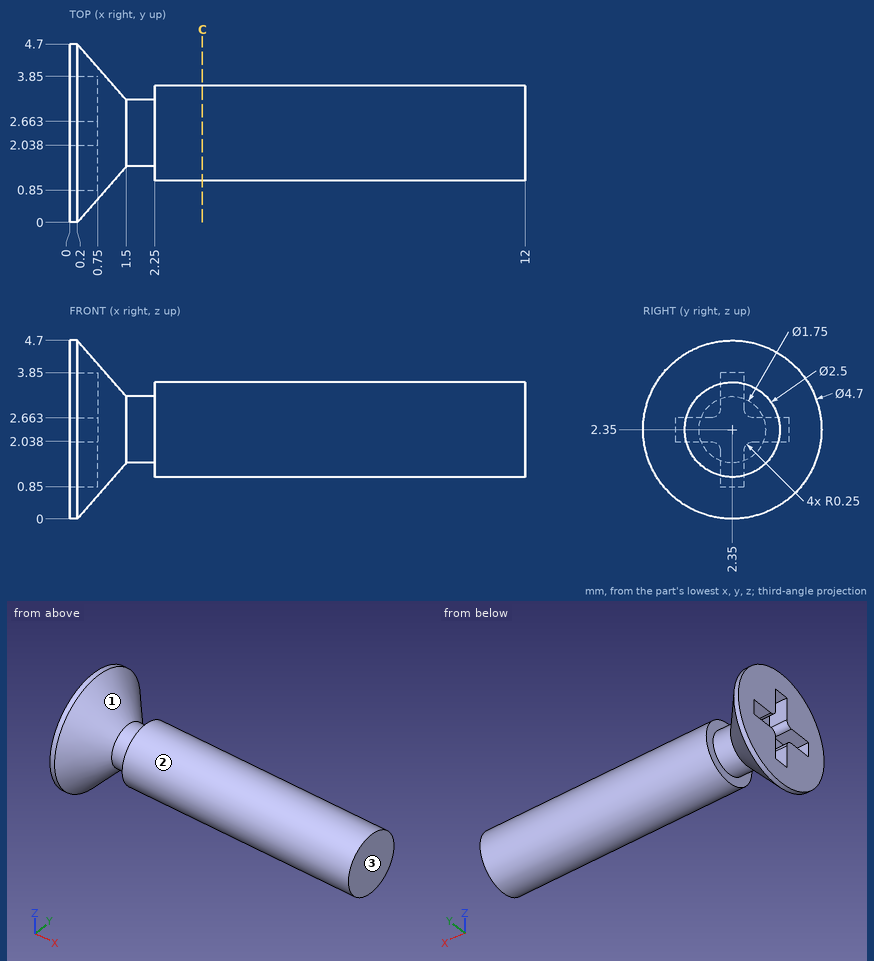
Study the drawing (mm; zero at the part's minimum x, y, z) and answer. A direction names the side the tool comes from. Round coordinates to 2 decimals unless told otherwise and drop trailing zeros. Loops run counter-clockwise (first coordinate to the right, second up) from the corner with the lowest first, then second, coordinate; pieces in that order, holes last.
Q1. Which of the six approach directions +Z, -Z, +X, -X, +Y, -Y give full straight-line access (tool end or side, diameter ignored) to the marked faces 1, 2 and 3?
Q2. Find the intervals of material crossed by line 1 (X direction, y = 1.55, z = 1.5); line 2 (Z direction, x = 1.75, y = 2.4); line 3 (X direction, y = 1.05, z = 1.8) (1 decimal), in increasing order.
Q3. Section C-C, the plane x = 3.5 is taken. Determine the outline of the cut face in (y, z).
Q4. Given pin 1 Ø2 at (x, y) = (3.5, 4) entering from -Z; pin 2 Ø0.8 at (x, y) = (0.5, 3.5) entering from -Z; pin 3 Ø0.5 at (x, z) = (0.5, 2.5) entering from +Y, each flat-ended and moving along its own axis, determine where each tip first touches the part or whether it passes through.
Completed:
1. face 1: none
1. face 2: +X
1. face 3: +Z, -Z, +X, +Y, -Y
2. line 1: x = 0 to 1.24, 2.25 to 12
2. line 2: z = 1.48 to 3.22
2. line 3: x = 0 to 1
3. outline: circle Ø2.5 at (2.35, 2.35)
4. pin 1: stops at z = 1.28
4. pin 2: stops at z = 0.17
4. pin 3: stops at y = 4.64
